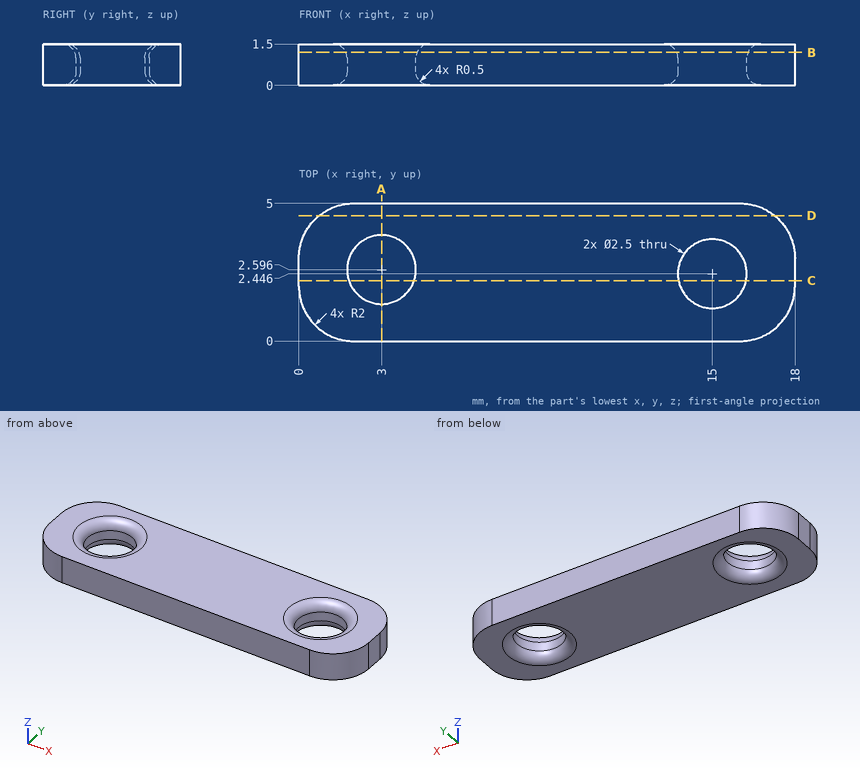
The figure shows three views and two pictorial views of one solid part (mm, origin at its lowest corner). Answer the questions. Round coordinates to 2 decimals unless told otherwise and drop trailing zeros. Write each loop counter-clockwise with the first axis right and the second up, starting at its lowest first coordinate (ties: lowest second). Pieces come first, ordered by that corner, then holes. Notation, with made-up numbers: M 43,-33.5 L 97,-33.5 A6 ccw 97,-28.5 Z; hole C -38.5,10 d1. An arc over 180 degrees is marked long. Write each question's results on one line, items separated by ' | '. Start each with the question number.
(1) This flat-tipped pin is pushed along its axis until it touches: P1, Ø1.5, axis at x = 15, y = 2.45, coming from the -Z side. Where does it stop, or does it pass through?
(2) The part is cut by section A-A, the plane x = 3. Write down the section's boundary in (y, z).
(3) The part is cut by section B-B, the plane z = 1.2. Write down the section's boundary in (x, y) (1 decimal).
(4) Find the intervals of material crossed by line 1 (Y direction, x = 3, z = 0.9); line 2 (Y direction, x = 15.5, z = 1.3); line 3 (X direction, y = 2.95, z = 0.9) (1 decimal), in increasing order.
(5) The part is cut by section C-C, the plane y = 2.2. Give the number of separate pieces and of enclosed holes in the cut face.
(6) The part is cut by section D-D, the plane y = 4.55. Write down the section's boundary in (x, z).
Worked answers:
1) P1: passes through
2) outline: M 0,0 L 0.85,0 A0.5 ccw 1.35,0.5 L 1.35,1 A0.5 ccw 0.85,1.5 L 0,1.5 Z; M 3.85,0.5 A0.5 ccw 4.35,0 L 5,0 L 5,1.5 L 4.35,1.5 A0.5 ccw 3.85,1 Z
3) outline: M 0,2 A2 ccw 2,0 L 16,0 A2 ccw 18,2 L 18,3 A2 ccw 16,5 L 2,5 A2 ccw 0,3 Z; hole C 3,2.6 d2.6; hole C 15,2.4 d2.6
4) line 1: y = 0 to 1.35, 3.85 to 5 | line 2: y = 0 to 1.19, 3.7 to 5 | line 3: x = 0 to 1.8, 4.2 to 13.9, 16.1 to 18
5) separate pieces: 3 | enclosed holes: 0
6) outline: M 0.74,0 L 17.26,0 L 17.26,1.5 L 0.74,1.5 Z
